Can you work these out from the drawing? Everything is in mm from the part's minimum corner. A direction names the side the tool comes from. Give positions to 0.01 mm unless a question says otherwise; leave off trailing zeros. Write each loop counter-clockwise with the first axis right and the second up, starting at its lowest first coordinate (ties: lowest second). Pieces come first, ordered by that corner, then holes. Notation, with made-up numbers: (-8, 79) - (30, 79) arc R14 ccw to (30, 100) - close; hole circle Ø9 at (42, -33.75). An arc over 180 degrees is marked (long way). Use a Markdown table: item, result.
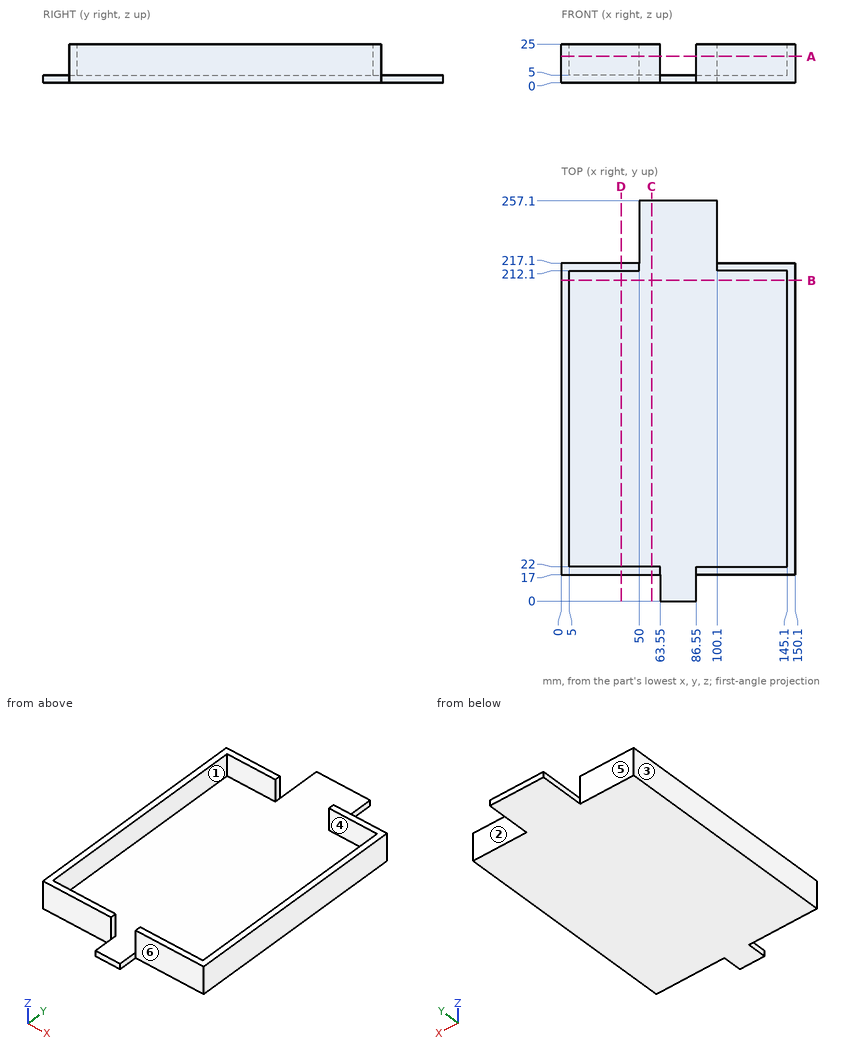
Item 1: Will these pins go through, and if not, where does the flat tip stop? pin 1 Ø2.5 at (y, z) = (8.5, 3.5) entering from -X; pin 2 Ø3 at (x, z) = (30, 17) entering from +Y; pin 3 Ø5 at (x, y) = (31.5, 128.5) entering from -Z; pin 4 Ø6 at (x, z) = (124.5, 7.5) entering from -Y.
Values:
| item | result |
|---|---|
| pin 1 | stops at x = 63.55 |
| pin 2 | stops at y = 217.1 |
| pin 3 | stops at z = 0 |
| pin 4 | stops at y = 17 |
Item 2: If we section it at C-C, the plane x = 58: Write out the boundary of the cut face in (y, z).
Values:
| item | result |
|---|---|
| outline | (17, 0) - (257.1, 0) - (257.1, 5) - (22, 5) - (22, 25) - (17, 25) - close |
Item 3: If we section it at D-D, the plane x = 38.5: Write out the boundary of the cut face in (y, z), plus the area to 3 significant figures.
Values:
| item | result |
|---|---|
| outline | (17, 0) - (217.1, 0) - (217.1, 25) - (212.1, 25) - (212.1, 5) - (22, 5) - (22, 25) - (17, 25) - close |
| area | 1,200 mm2 |
Item 4: Thinking about a two-plate mould opening in X: for the marked faces 1, 2 and 3, which applies, +X half, -X half, draft (parallel to the pull), parting line (faces both ways), or undercut?
Values:
| item | result |
|---|---|
| face 1 | undercut |
| face 2 | draft |
| face 3 | -X half |
Item 5: For the marked faces 4, 5 and 6, which set-ups out of +Z, -Z, +X, -X, +Y, -Y let a thin tool reach every point of the face, with its end or its side?
Values:
| item | result |
|---|---|
| face 4 | +Z |
| face 5 | +Z, -Z, -X, +Y |
| face 6 | +Z, -Z, +X, -Y |
Item 6: If we section it at A-A, the plane z = 17: Write out the boundary of the cut face in (x, y).
Values:
| item | result |
|---|---|
| outline | (0, 17) - (63.55, 17) - (63.55, 22) - (5, 22) - (5, 212.1) - (50, 212.1) - (50, 217.1) - (0, 217.1) - close; (86.55, 17) - (150.1, 17) - (150.1, 217.1) - (100.1, 217.1) - (100.1, 212.1) - (145.1, 212.1) - (145.1, 22) - (86.55, 22) - close |
Item 7: I need wall thicknesses on line 1 along X through (y, z) = (51.5, 10.25); line 2 along Y through (x, z) = (122, 18.5); line 3 along Z through (x, y) = (46, 207). Which ranges of each line are inside material? Lowest first, please. Write a range as [from, to].
Values:
| item | result |
|---|---|
| line 1 | x = [0, 5], [145.1, 150.1] |
| line 2 | y = [17, 22], [212.1, 217.1] |
| line 3 | z = [0, 5] |
Item 8: If we section it at B-B, the plane y = 206: Write out the boundary of the cut face in (x, z).
Values:
| item | result |
|---|---|
| outline | (0, 0) - (150.1, 0) - (150.1, 25) - (145.1, 25) - (145.1, 5) - (5, 5) - (5, 25) - (0, 25) - close |
